from build123d import *

# Parameters (mm, degrees)
PAD009_DEPTH = 9.5


with BuildPart() as part:
    # Sketch018 → Pad009 (new body)
    with BuildSketch(Plane.XY.offset(-1)):
        with BuildLine():
            Line((-4, 3.858899), (4, 3.858899))
            Line((4, 3.858899), (2.94356, -1.02822))
            ThreePointArc((0.5, -3), (2.069944, -2.445578), (2.94356, -1.02822))
            Line((0.5, -3), (-0.5, -3))
            ThreePointArc((-2.94356, -1.02822), (-2.069944, -2.445578), (-0.5, -3))
            Line((-2.94356, -1.02822), (-4, 3.858899))
        make_face()
    extrude(amount=-PAD009_DEPTH)


solid = part.part
The listing builds one solid part. Answer for the finished solid, in the listing's coordinates (mm). Coordinates: 2 decimals unless noted, no trailing zeros. Write each loop counter-clockwise with the first axis right and the second up, starting at its lowest first coordinate (ties: lowest second). Pieces come first, ordered by that corner, then holes. Notation, with made-up numbers: (21, 44.5) - (60, 44.5) arc R12 ccw to (60, 61.5) - close; hole circle Ø3 at (84.25, 88). An arc over 180 degrees is marked (long way). Return JSON: item names as keys, results as strings.
1. The part is cut by section B-B on x = 2. Determine the outline of the cut face in (y, z), then the cut area to 3 significant figures.
Final values:
{"outline": "(-2.5, -10.5) - (3.86, -10.5) - (3.86, -1) - (-2.5, -1) - close", "area": "60.4 mm^2"}
2. Each of these flat-tipped pins is pushed along its axis until it touches: pin 1 Ø2 at (y, z) = (2.5, -9.5) entering from -X; pin 2 Ø2 at (y, z) = (0, -5) entering from +X; pin 3 Ø4 at (y, z) = (1, -5.5) entering from -X. Where does it stop, or does it pass through?
Final values:
{"pin 1": "x = -3.92", "pin 2": "x = 3.38", "pin 3": "x = -3.81"}
3. The part is cut by section A-A on z = -6. Determine the outline of the cut face in (x, y).
Final values:
{"outline": "(-4, 3.86) - (-2.94, -1.03) arc R2.5 ccw to (-0.5, -3) - (0.5, -3) arc R2.5 ccw to (2.94, -1.03) - (4, 3.86) - close"}
4. The part is cut by section C-C on y = 2.75. Determine the outline of the cut face in (x, z), then the cut area to 3 significant figures.
Final values:
{"outline": "(-3.76, -10.5) - (3.76, -10.5) - (3.76, -1) - (-3.76, -1) - close", "area": "71.4 mm^2"}
5. Consider line 1 along Y through (x, z) = (-1.5, -8.25); line 2 along Y through (x, z) = (2, -4.75); line 3 along X through (y, z) = (-1.75, -4.5). Determine where each line is inside the solid, lowest interval first.
Final values:
{"line 1": "-2.79 to 3.86", "line 2": "-2.5 to 3.86", "line 3": "-2.67 to 2.67"}
